Study the drawing (mm; zero at the part's minimum x, y, z) and answer. Coordinates: 2 decimals unless noted, no trailing zeros. Order: outer loops, then holes, each group sorted by start corner. A loop starts at its lowest first (then second) coordinate and runs counter-clockwise, first axis right, second up. Notation, with made-up numbers: M -15.75,-23 L -11.75,-23 A22 ccw -11.75,-4 Z; hole C 46.5,77 d11. An arc over 180 degrees is marked long. Use a Markdown table: item, result. Add a question column.
1) Find the intervals of material crossed by probe 1 along Z at (x, y) = (5, 23) (1 decimal); probe 2 along Y at (x, z) = (5.5, 10.5); probe 3 along Y at (x, z) = (6, 32), in increasing order. Write a range as [from, to].
2) Find section B-B on y = 7.5. Write down the section's boundary in (x, z).
3) Find section C-C on z = 20. Write down the section's boundary in (x, y).
4) Each of these flat-tipped pins is pushed along its axis until it touches: pin 1 Ø2 at (x, y) = (16, 16.5) entering from -Z; pin 2 Ø6 at (x, y) = (14, 6.5) entering from +Z (1 decimal); pin 3 Ø3 at (x, y) = (13.5, 23) entering from +Z. Where does it stop, or does it pass through?
5) Find section A-A on x = 16.5. Write down the section's boundary in (y, z), plus the area to 3 significant figures.
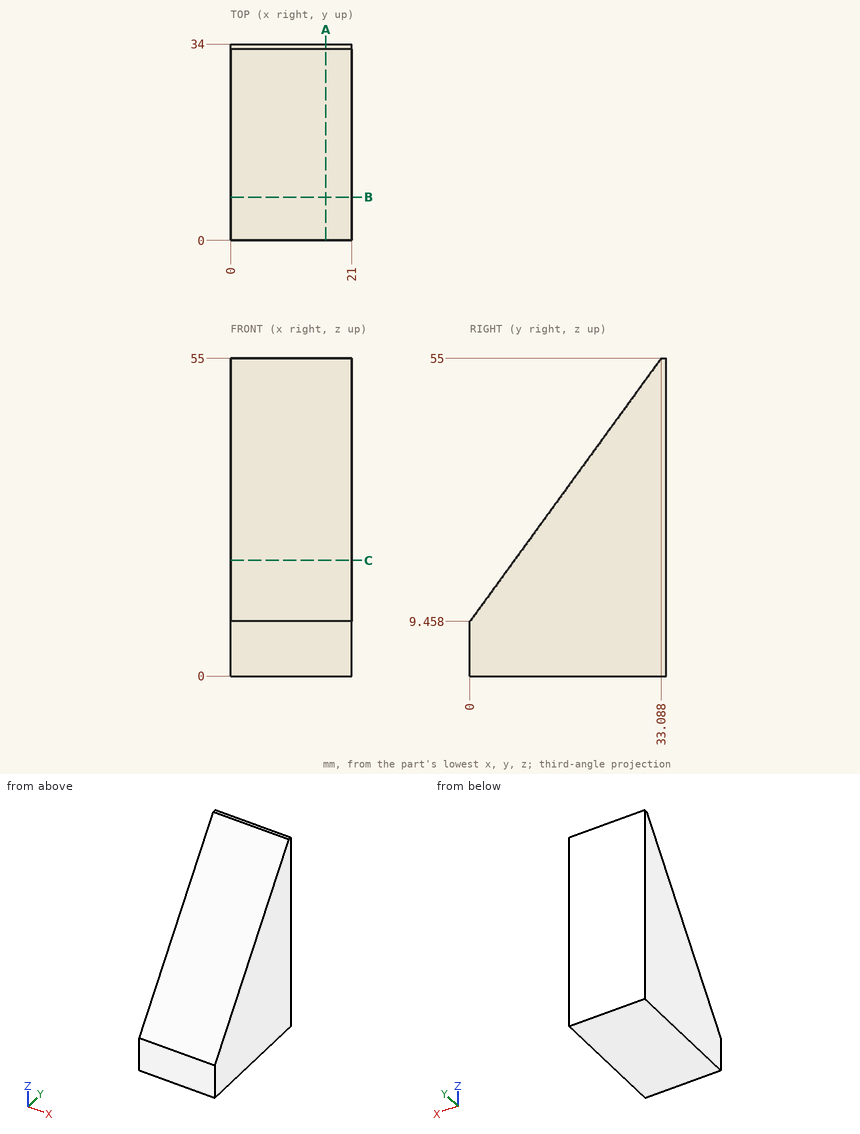
Check result:
| question | item | result |
|---|---|---|
| 1 | probe 1 | z = [0, 41.1] |
| 1 | probe 2 | y = [0.76, 34] |
| 1 | probe 3 | y = [16.38, 34] |
| 2 | outline | M 0,0 L 21,0 L 21,19.78 L 0,19.78 Z |
| 3 | outline | M 0,7.66 L 21,7.66 L 21,34 L 0,34 Z |
| 4 | pin 1 | stops at z = 0 |
| 4 | pin 2 | stops at z = 22.5 |
| 4 | pin 3 | stops at z = 43.18 |
| 5 | outline | M 0,0 L 34,0 L 34,55 L 33.09,55 L 0,9.46 Z |
| 5 | area | 1,120 mm2 |
